Autodesk Inventor part; units mm, degrees
ref_plane "YZ Plane" through (0, 0, 0) normal (1, 0, 0) x (0, 1, 0)
ref_plane "XZ Plane" through (0, 0, 0) normal (0, 1, 0) x (-1, 0, 0)
ref_plane "XY Plane" through (0, 0, 0) normal (0, 0, 1) x (1, 0, 0)
sketch "Sketch1" plane through (0, 0, 0) normal (0, 1, 0) x (-1, 0, 0)
  line L0 (34.4615, 64) -> (34.4615, -64)
  line L1 (-34.4615, -64) -> (-34.4615, 64)
  line L2 (-34.4615, 64) -> (34.4615, -64) construction
  line L3 (34.4615, 64) -> (-34.4615, -64) construction
  arc A0 (-34.4615, -64) -> (34.4615, -64) centre (0, -1.4222) ccw
  arc A1 (34.4615, 64) -> (-34.4615, 64) centre (0, 1.4222) ccw
  point P0 (0, 0)
  dimension "d1" = 128
extrude "taban" add sketch "Sketch1" along normal blind 3
sketch "Sketch2" plane through (0, 3, 0) normal (0, 1, 0) x (1, 0, 0)
  circle A0 centre (0, 30) radius 12.5
  circle A1 centre (0, -30) radius 12.5
extrude "cam" cut sketch "Sketch2" against normal blind 3
sketch "Sketch3" plane through (34.4615, 0, 64) normal (1, 0, 0) x (0, 0, -1)
  line L0 (12, 3) -> (31, 3)
  line L1 (31, 3) -> (31, 0)
  line L2 (31, 0) -> (12, 0)
  line L3 (12, 0) -> (12, 3)
  line L4 (118, 3) -> (99, 3)
  line L5 (99, 3) -> (99, 0)
  line L6 (99, 0) -> (118, 0)
  line L7 (118, 0) -> (118, 3)
extrude "sikigecme" add sketch "Sketch3" along normal blind 3
chamfer "Chamfer1" distance 1 angle 45 4 edges at (-12.5, 0, -30) (-12.5, 0, 30) (-12.5, 3, 30) (-12.5, 3, -30)
properties part number "VR_Cam_Kismi_3DPrint"
Work out the finished part from the listing and answer in its coordinate system (mm). A direction names the side the tool comes from. Coordinates: 2 decimals unless noted, no trailing zeros. Loops run counter-clockwise (first coordinate to the right, second up) from the corner with the lowest first, then second, coordinate; pieces in that order, holes last. Notation, with made-up numbers: (-9.5, 44) -> (49.5, 44) arc R28 cw to (49.5, 64) -> close; hole circle Ø4 at (83.25, 44.25). An arc over 180 degrees is marked (long way). Answer as CSV lines item,"result".
1) For a pull along Z with two mould halves and no side action, classify faces 1 (the face through (6.72, 1.51, -40.54)), 2 (the face through (-0.5, 1.48, -72.86)), 3 (the face through (36, 1, 52)), 4 (the face through (-2.71, 1.507, 42.203)) as released by +Z, released by -Z, zero draft, split by the parting line, or undercut.
A:
face 1,"undercut"
face 2,"released by -Z"
face 3,"released by +Z"
face 4,"undercut"
2) The part is cut by section B-B (z = 30). Give the vertices of the cut face in (x, y).
A:
outline,"(-34.46, 0) -> (-13.5, 0) -> (-12.5, 1) -> (-12.5, 2) -> (-13.5, 3) -> (-34.46, 3) -> close; (12.5, 1) -> (13.5, 0) -> (34.46, 0) -> (34.46, 3) -> (13.5, 3) -> (12.5, 2) -> close"
3) Flat-ended cylindrical pins translate along their axes: pin 1 (0.9 mm diameter, centred on y = 1, z = 58.5, fed in from +X); pin 2 (10 mm diameter, centred on x = 0, z = 35.5, fed in from +Y); pin 3 (8 mm diameter, centred on x = -2.5, z = -17, fed in from -Y). Find the tip coordinate at first contact, or state that the pin passes through.
A:
pin 1,"stops at x = 34.46"
pin 2,"passes through"
pin 3,"stops at y = 0"
4) The part is cut by section A-A (x = 0). Give the vertices of the cut face in (y, z).
A:
outline,"(0, -72.86) -> (3, -72.86) -> (3, -43.5) -> (2, -42.5) -> (1, -42.5) -> (0, -43.5) -> close; (0, -16.5) -> (1, -17.5) -> (2, -17.5) -> (3, -16.5) -> (3, 16.5) -> (2, 17.5) -> (1, 17.5) -> (0, 16.5) -> close; (0, 43.5) -> (1, 42.5) -> (2, 42.5) -> (3, 43.5) -> (3, 72.86) -> (0, 72.86) -> close"
5) Straight lines are drawn through the part: probe 1 along X at (y, z) = (1.7, 30); probe 2 along Z at (x, y) = (8.5, 2.6); probe 3 along Z at (x, y) = (5.5, 0.75). For each, find the intervals that lie inside material, in ascending order.
A:
probe 1,"x = -34.46 to -12.5, 12.5 to 34.46"
probe 2,"z = -72.35 to -39.97, -20.03 to 20.03, 39.97 to 72.35"
probe 3,"z = -72.65 to -41.5, -18.5 to 18.5, 41.5 to 72.65"
6) For faces 5 (the face through (34.462, 1, -59)), 6 (the face through (37.462, 2, -44)), 7 (the face through (34.462, 1, 58)), 8 (the face through (36, 2, 33)), determine the directions among +Z, -Z, +X, -X, +Y, -Y from which every point of the face is accessible in a straight line to the end or side of a thin tool.
A:
face 5,"-Z, +X, +Y, -Y"
face 6,"+Z, -Z, +X, +Y, -Y"
face 7,"+Z, +X, +Y, -Y"
face 8,"+X, +Y, -Y"
7) The part is cut by section D-D (x = 22). Give the vertices of the cut face in (y, z).
A:
outline,"(0, -69.39) -> (3, -69.39) -> (3, 69.39) -> (0, 69.39) -> close"
8) The part is cut by section C-C (z = 7). Give the vertices of the cut face in (x, y), and give its area (3 significant figures).
A:
outline,"(-34.46, 0) -> (34.46, 0) -> (34.46, 3) -> (-34.46, 3) -> close"
area,"207 mm²"
